Answer from the drawing. Dimensions are ordinates in mm from the lowest x, y and z of the part. A direction names the side the tool comes from. Round coordinates to 2 decimals unless told otherwise and drop trailing zeros. Write each loop counter-clockwise with the first axis right and the second up, starting at its lowest first coordinate (ties: lowest second). Pieces come first, ordered by that corner, then holes. Notation, with made-up numbers: (63, 63.25) - (80, 63.25) arc R22 cw to (80, 72.25) - close; hole circle Ø10 at (-15, 41.5). An arc over 180 degrees is marked (long way). Answer as a JSON object with one key per item and string values.
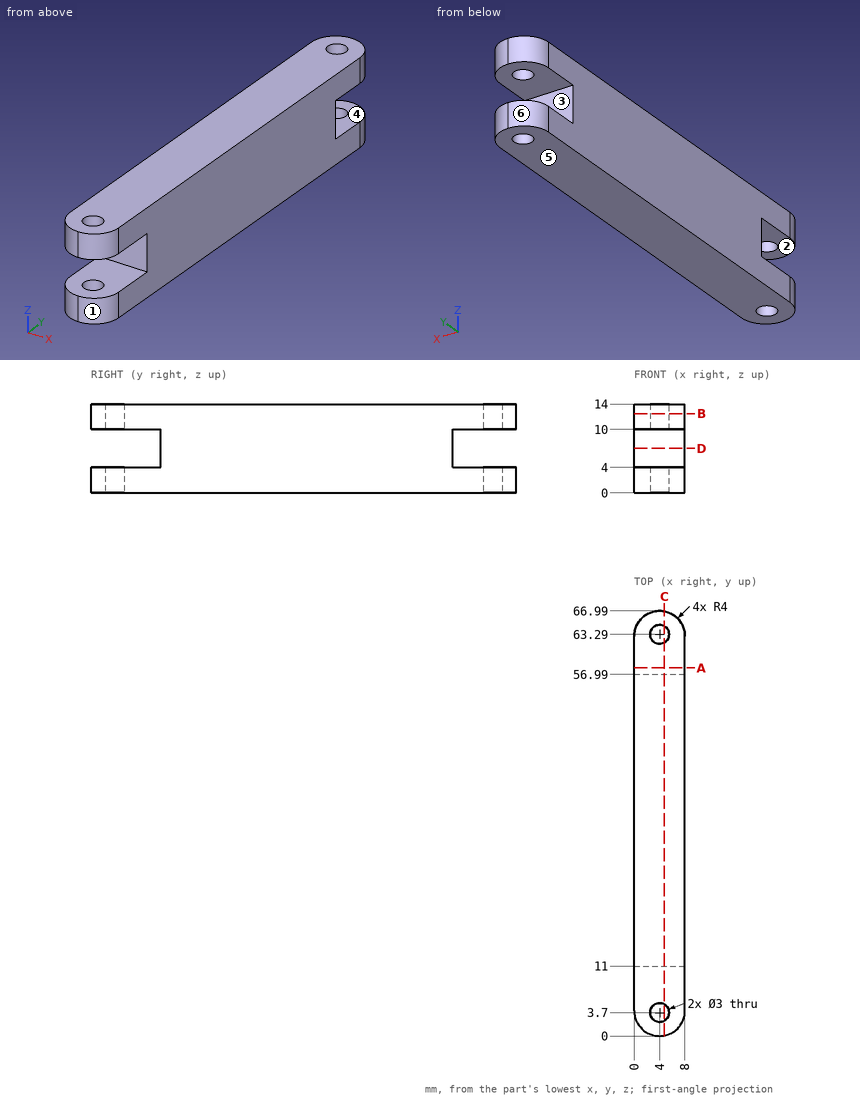
Item 1: For the marked faces 1, 2 and 3, determine the directions among +Z, -Z, +X, -X, +Y, -Y from which every point of the face is accessible in a straight line to the end or side of a thin tool.
Results found:
{"face 1": "+Z, -Z, +X, -Y", "face 2": "+X, -X, -Y", "face 3": "+X, -X, +Y"}
Item 2: Consider line 1 along Y through (x, z) = (4, 12.05); line 2 along Z through (x, y) = (6, 8); line 3 along Y through (x, z) = (2.25, 8). Determine where each line is inside the solid, lowest interval first.
Results found:
{"line 1": "0 to 2.2, 5.2 to 61.79, 64.79 to 66.99", "line 2": "0 to 4, 10 to 14", "line 3": "11 to 56.99"}
Item 3: Determine the mould class of the marked faces 4, 5 and 6 for opening direction Z: pulls with the +Z half, pulls with the -Z half, needs draft (parallel to the pull), parting line crosses it, or undercut.
Results found:
{"face 4": "undercut", "face 5": "pulls with the -Z half", "face 6": "needs draft"}
Item 4: A cutting plane is placed at C-C (x = 4.75). Write down the section's boundary in (y, z), and give its area (3 significant figures).
Results found:
{"outline": "(0.07, 0) - (2.4, 0) - (2.4, 4) - (0.07, 4) - close; (0.07, 10) - (2.4, 10) - (2.4, 14) - (0.07, 14) - close; (5, 0) - (61.99, 0) - (61.99, 4) - (56.99, 4) - (56.99, 10) - (61.99, 10) - (61.99, 14) - (5, 14) - (5, 10) - (11, 10) - (11, 4) - (5, 4) - close; (64.59, 0) - (66.92, 0) - (66.92, 4) - (64.59, 4) - close; (64.59, 10) - (66.92, 10) - (66.92, 14) - (64.59, 14) - close", "area": "769 mm²"}
Item 5: A cutting plane is placed at B-B (z = 12.5). Give the number of separate pieces and of enclosed holes in the cut face, and give its area (3 significant figures).
Results found:
{"separate pieces": "1", "enclosed holes": "2", "area": "508 mm²"}
Item 6: A cutting plane is placed at D-D (z = 7). Write down the section's boundary in (x, y), and give its area (3 significant figures).
Results found:
{"outline": "(0, 11) - (8, 11) - (8, 56.99) - (0, 56.99) - close", "area": "368 mm²"}
Item 7: This flat-tipped pin is pushed along its axis until it touches: P1, Ø1, axis at x = 7, z = 3.5, coming from the +Y side. Where does it stop, or does it pass through?
Results found:
{"P1": "y = 66.11"}
Item 8: A cutting plane is placed at A-A (y = 58). Write down the section's boundary in (x, z).
Results found:
{"outline": "(0, 0) - (8, 0) - (8, 4) - (0, 4) - close; (0, 10) - (8, 10) - (8, 14) - (0, 14) - close"}
